Verification items for the finished model (mm, model axes). Face numbers are marked on the shaded views. A direction names the side the tool comes from. Give positions to 0.01 mm unless a question says otherwise; leave off trailing zeros. Loops run counter-clockwise (first coordinate to the right, second up) from the corner with the lowest first, then second, coordinate; pieces in that order, holes last. Notation, with made-up numbers: (32, 5.5) -> (66, 5.5) arc R19 cw to (66, 41.5) -> close; hole circle Ø5 at (-16.5, 89.25). An arc over 180 degrees is marked (long way). Answer in a Markdown table with one row per item. Add a question column.
Q1. Section check A-A on y = 0. Enter the section's corners in (x, z), and give its area (3 significant figures).
Q2. Section check D-D on z = -1. Enter the section's corners in (x, y), and give its area (3 significant figures).
Q3. Section check C-C on z = 4.25. Enter the section's corners in (x, y).
Q4. Set-up check for the marked faces 4 and 5: record each of +Z, -Z, +X, -X, +Y, -Y from which the full face is reachable in a straight line by a thin tool's end or side.
Q5. Release check for a two-part mould opening along Z. For the marked faces 1, 2 and 3 record: pulls with the +Z half, pulls with the -Z half, needs draft (parallel to the pull), parting line crosses it, or undercut.
Q6. Gauge pin test, flat ends, axial feed: P1, Ø1, axis at y = -4.5, z = 0.5, coming from the -X side; P2, Ø2, axis at y = 3, z = -3.5, coming from the +X side; P3, Ø3, axis at x = -5, z = 1.5, coming from the -Y side. Record the tip position at first contact, or that the pin passes through.
Q7. Material ranges on probe 1 along Y at (x, z) = (0, 1.5); probe 2 along Z at (x, y) = (-4.5, 8.25); probe 3 along Z at (x, y) = (-9, 3.5), recorded low to high.
```python
from build123d import *

# Parameters (mm, degrees)
SKETCH1_R           = 10
BOSS_EXTRUDE1_DEPTH = 5


with BuildPart() as part:
    # Sketch1 → Boss-Extrude1 (new body, symmetric)
    with BuildSketch(Plane.XY):
        Circle(SKETCH1_R)
    extrude(amount=BOSS_EXTRUDE1_DEPTH, both=True)

    # Sketch2 → Cut-Revolve1 (revolve, cut)
    with BuildSketch(Plane(origin=(0, 0, 0), x_dir=(1, 0, 0), z_dir=(0, 1, 0))):
        Polygon((10, 3), (8.178550696, 1.948385754), (8.178550696, -1.948385754), (10, -3), align=None)
    revolve(axis=Axis((0, 0, -6.38791657), (0, 0, 1)), mode=Mode.SUBTRACT)


solid = part.part
```
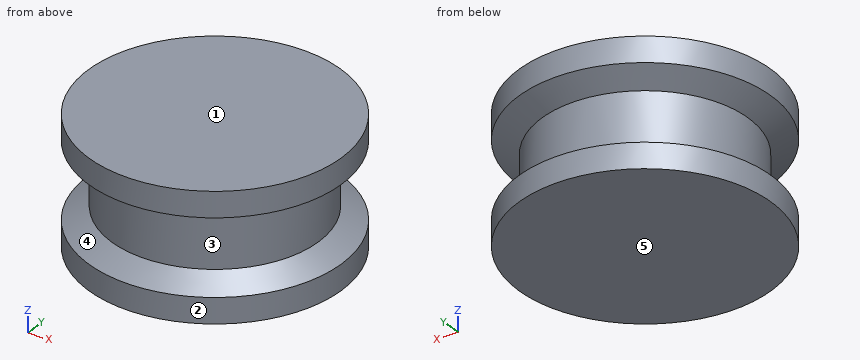
Taken from the geometry:
| question | item | result |
|---|---|---|
| 1 | outline | (-10, -5) -> (10, -5) -> (10, -3) -> (8.18, -1.95) -> (8.18, 1.95) -> (10, 3) -> (10, 5) -> (-10, 5) -> (-10, 3) -> (-8.18, 1.95) -> (-8.18, -1.95) -> (-10, -3) -> close |
| 1 | area | 182 mm² |
| 2 | outline | circle Ø16.36 at (0, 0) |
| 2 | area | 210 mm² |
| 3 | outline | circle Ø20 at (0, 0) |
| 4 | face 4 | none |
| 4 | face 5 | -Z, +X, -X, +Y, -Y |
| 5 | face 1 | pulls with the +Z half |
| 5 | face 2 | needs draft |
| 5 | face 3 | undercut |
| 6 | P1 | stops at x = -7.13 |
| 6 | P2 | stops at x = 9.8 |
| 6 | P3 | stops at y = -8.77 |
| 7 | probe 1 | y = -8.18 to 8.18 |
| 7 | probe 2 | z = -5 to -2.65, 2.65 to 5 |
| 7 | probe 3 | z = -5 to -2.8, 2.8 to 5 |
